Verification items for the finished model (mm, model axes). A direction names the side the tool comes from. Coordinates: 2 decimals unless noted, no trailing zeros. Order: outer loops, then holes, each group sorted by start corner. A loop starts at its lowest first (then second) coordinate and runs counter-clockwise, first axis right, second up. Notation, with made-up numbers: (17.5, -38) -> (73.5, -38) arc R8 cw to (73.5, -33) -> close; hole circle Ø7 at (75.5, -5). An arc over 180 degrees is marked (long way). Write item = value, one per line. Start each with the question number.
1. Cross-section at A-A on y = 5.5. Record the cut outline in (x, z), plus the area to 3 significant figures.
2. Set-up check for faces 1 (the cylindrical face through (-103.4, 31.3, -92.2)), 2 (the flat face through (0, 17, -66)): record each of +Z, -Z, +X, -X, +Y, -Y from which the full face is reachable in a straight line by a thin tool's end or side.
3. Go/stop test with a flat-tipped pin: P1, Ø1.8, axis at x = -102.5, z = -35, coming from the -Y side. Record where the tip stops, or that it passes through.
4. Cross-section at B-B on z = -75.5. Record the cut outline in (x, y), plus the area to 3 significant figures.
5. Cross-section at C-C on x = -46.5. Record the cut outline in (y, z).
6. Thickness scan on line 1 along X through (y, z) = (34, -36); line 2 along Z through (x, y) = (-101, 33); line 3 along Z through (x, y) = (-76.5, 2). Record the ranges inside material, lowest first. Write a range as from..to.
7. Release check for a two-part mould opening along Z. For faces 3 (the flat face through (-122, 17, -130)), 4 (the flat face through (-118, 35, -64)), 5 (the flat face through (-118, 17, 0)), 6 (the flat face through (-2.5, 16, -71)) record: +Z half, -Z half, draft (parallel to the pull), parting line (faces both ways), or undercut.
Autodesk Inventor part; units mm, degrees
ref_plane "YZ Plane" through (0, 0, 0) normal (1, 0, 0) x (0, 1, 0)
ref_plane "XZ Plane" through (0, 0, 0) normal (0, 1, 0) x (-1, 0, 0)
ref_plane "XY Plane" through (0, 0, 0) normal (0, 0, 1) x (1, 0, 0)
sketch "Sketch1" plane through (0, 0, 0) normal (0, 1, 0) x (-1, 0, 0)
  line L0 (0, 0) -> (240, 0)
  line L1 (240, 0) -> (240, -130)
  line L2 (240, -130) -> (0, -130)
  line L3 (0, -130) -> (0, 0)
  dimension "d0" = 130
  dimension "d1" = 240
extrude "Extrusion1" add sketch "Sketch1" along normal blind 35
sketch "Sketch2" plane through (0, 0, 0) normal (0, -1, 0) x (1, 0, 0)
  line L0 (-5, -111) -> (-105, -111) construction
  line L1 (-105, -111) -> (-105, -32) construction
  line L2 (-105, -32) -> (-5, -32) construction
  line L3 (-5, -32) -> (-5, -111) construction
  line L4 (-15, -94) -> (-101, -94) construction
  line L5 (-101, -94) -> (-101, -36) construction
  line L6 (-101, -36) -> (-15, -36) construction
  line L7 (-15, -36) -> (-15, -94) construction
  line L8 (-103.25, -76.2) -> (-99.35, -76.2) construction
  line L9 (-99.35, -76.2) -> (-99.35, -53.8) construction
  line L10 (-99.35, -53.8) -> (-103.25, -53.8) construction
  line L11 (-103.25, -53.8) -> (-103.25, -76.2) construction
  line L12 (0, 0) -> (-240, 0) construction
  line L13 (-240, -130) -> (0, -130) construction
  line L14 (-2.5, -113.5) -> (-107.5, -113.5)
  line L15 (-107.5, -113.5) -> (-107.5, -29.5)
  line L16 (-107.5, -29.5) -> (-2.5, -29.5)
  line L17 (-2.5, -29.5) -> (-2.5, -113.5)
  line L18 (0, -130) -> (0, 0)
  dimension "d5" = 100
  dimension "d6" = 86
  dimension "d7" = 58
  dimension "d8" = 79
  dimension "d9" = 4
  dimension "d10" = 4
  dimension "d12" = 22.4
  dimension "d13" = 17.8
  dimension "d14" = 130
  dimension "d16" = 53.8
  dimension "d17" = 3.9
  dimension "d18" = 1.75
  dimension "d19" = 105
  dimension "d20" = 2.5
  dimension "d21" = 84
  dimension "d22" = 2.5
  dimension "d25" = 2.5
extrude "Extrusion2" cut sketch "Sketch2" against normal blind 32.5
sketch "Sketch3" plane through (0, 32.5, 0) normal (0, -1, 0) x (1, 0, 0)
  circle A0 centre (-15, -94) radius 3
  circle A1 centre (-101, -94) radius 3
  circle A2 centre (-15, -36) radius 3
  circle A3 centre (-101, -36) radius 3
  point P0 (0, 0)
  dimension "d26" = 6
  dimension "d27" = 6
  dimension "d28" = 6
  dimension "d29" = 6
extrude "Extrusion3" add sketch "Sketch3" along normal blind 1.5
fillet "Fillet1" radius 1 4 edges at (-18, 32.5, -94) (-104, 32.5, -94) (-18, 32.5, -36) (-104, 32.5, -36)
sketch "Sketch4" plane through (-15, 31, -94) normal (0, -1, 0) x (1, 0, 0)
  circle A0 centre (0, 0) radius 3 construction
  circle A1 centre (0, 58) radius 3 construction
  circle A2 centre (-86, 58) radius 3 construction
  circle A3 centre (-86, 0) radius 3 construction
  circle A4 centre (0, 0) radius 3 construction
  circle A5 centre (-86, 58) radius 4 construction
  point P0 (15, 94)
hole "Hole1" at (-15, 31, -94) at (-15, 31, -36) at (-101, 31, -36) at (-101, 31, -94) direction (0, 1, 0) diameter 2.4 depth 4
equation "\"d10\" = d9"
equation "\"d16\" = -0.5 * d12 + 0.5 * d14"
equation "\"d22\" = -0.5 * d8 + 0.5 * d21"
equation "\"d25\" = -0.5 * d5 + 0.5 * d19"
properties part number "Chassis"
Worked out:
q1.outline = (-240, -130) -> (0, -130) -> (0, 0) -> (-240, 0) -> close; hole (-107.5, -113.5) -> (-2.5, -113.5) -> (-2.5, -29.5) -> (-107.5, -29.5) -> close
q1.area = 22,400 mm²
q2.face_1 = -Y
q2.face_2 = +Z, -Z, +X, +Y, -Y
q3.P1 = 31
q4.outline = (-240, 0) -> (-107.5, 0) -> (-107.5, 32.5) -> (-2.5, 32.5) -> (-2.5, 0) -> (0, 0) -> (0, 35) -> (-240, 35) -> close
q4.area = 4,990 mm²
q5.outline = (0, -130) -> (35, -130) -> (35, 0) -> (0, 0) -> (0, -29.5) -> (32.5, -29.5) -> (32.5, -113.5) -> (0, -113.5) -> close
q6.line_1 = -240..-102.2, -99.8..-16.2, -13.8..0
q6.line_2 = -130..-95.2, -92.8..-37.2, -34.8..0
q6.line_3 = -130..-113.5, -29.5..0
q7.face_3 = -Z half
q7.face_4 = draft
q7.face_5 = +Z half
q7.face_6 = undercut
